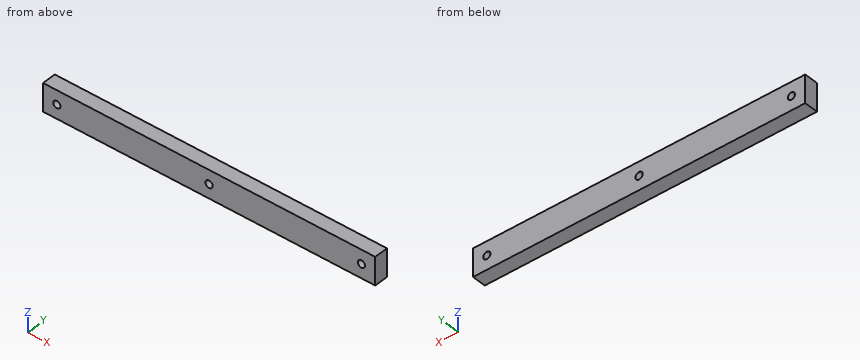
from build123d import *

# Parameters (mm, degrees)
SKETCH1_W                      = 304.8
SKETCH1_H                      = 25.4
BOSS_EXTRUDE1_DEPTH            = 12.7
M6_CLEARANCE_HOLE1_D           = 6.6
M6_CLEARANCE_HOLE1_CSINK_D     = 6.65
M6_CLEARANCE_HOLE1_CSINK_ANGLE = 90


with BuildPart() as part:
    # Sketch1 → Boss-Extrude1 (new body)
    with BuildSketch(Plane(origin=(0, 0, 0), x_dir=(1, 0, 0), z_dir=(0, 1, 0))):
        Rectangle(SKETCH1_W, SKETCH1_H)
    extrude(amount=BOSS_EXTRUDE1_DEPTH)

    # M6 Clearance Hole1 (through all)
    with Locations(Plane.ZX.offset(12.7)):
        with Locations((0, 0), (0, -139.7), (0, 139.7)):
            CounterSinkHole(M6_CLEARANCE_HOLE1_D / 2, M6_CLEARANCE_HOLE1_CSINK_D / 2, counter_sink_angle=M6_CLEARANCE_HOLE1_CSINK_ANGLE)


solid = part.part
Geometry check sheet. Reference: the model listing, model coordinates, mm. Give positions to 0.01 mm unless a question says otherwise; leave off trailing zeros. Loops run counter-clockwise (first coordinate to the right, second up) from the corner with the lowest first, then second, coordinate; pieces in that order, holes last. Notation, with made-up numbers: (3.5, 51.5) -> (51.5, 51.5) arc R8 cw to (51.5, 64.5) -> close; hole circle Ø7 at (29.25, -5). An arc over 180 degrees is marked (long way). Answer in a Markdown table with one row per item. Add a question column.
1) Cross-section at A-A on x = 0. Record the boundary of the cut face in (y, z) (3 decimals).
2) Cross-section at B-B on z = 0. Record the boundary of the cut face in (x, y) (3 decimals), and give its area (3 significant figures).
3) Material ranges on probe 1 along X at (y, z) = (3, 0); probe 2 along Z at (x, y) = (0, 5.25), recorded low to high. Write a range as from..to.
4) Gauge pin test, flat end, axial feed: P1, Ø6, axis at x = -139.7, z = 0, coming from the -Y side. Record the tip position at first contact, or that the pin passes through.
Outcome:
| question | item | result |
|---|---|---|
| 1 | outline | (0, -12.7) -> (12.7, -12.7) -> (12.7, -3.325) -> (12.675, -3.3) -> (0, -3.3) -> close; (0, 3.3) -> (12.675, 3.3) -> (12.7, 3.325) -> (12.7, 12.7) -> (0, 12.7) -> close |
| 2 | outline | (-152.4, 0) -> (-143, 0) -> (-143, 12.675) -> (-143.025, 12.7) -> (-152.4, 12.7) -> close; (-136.4, 0) -> (-3.3, 0) -> (-3.3, 12.675) -> (-3.325, 12.7) -> (-136.375, 12.7) -> (-136.4, 12.675) -> close; (3.3, 0) -> (136.4, 0) -> (136.4, 12.675) -> (136.375, 12.7) -> (3.325, 12.7) -> (3.3, 12.675) -> close; (143, 0) -> (152.4, 0) -> (152.4, 12.7) -> (143.025, 12.7) -> (143, 12.675) -> close |
| 2 | area | 3,620 mm^2 |
| 3 | probe 1 | x = -152.4..-143, -136.4..-3.3, 3.3..136.4, 143..152.4 |
| 3 | probe 2 | z = -12.7..-3.3, 3.3..12.7 |
| 4 | P1 | passes through |
